from build123d import *

# Parameters (mm, degrees)
CROQUIS1_W              = 41
CROQUIS1_H              = 23.5
CROQUIS1_R              = 5.3
SALIENTE_EXTRUIR1_DEPTH = 3
CROQUIS3_W              = 41
CROQUIS3_H              = 3
SALIENTE_EXTRUIR2_DEPTH = 27
CROQUIS4_R              = 1.8
SALIENTE_EXTRUIR3_DEPTH = 3
CROQUIS5_W              = 8.5
CROQUIS5_H              = 3
SALIENTE_EXTRUIR4_DEPTH = 27
CROQUIS6_W              = 38
CROQUIS6_H              = 3
SALIENTE_EXTRUIR5_DEPTH = 12
CORTAR_EXTRUIR3_REACH   = 54.868
CROQUIS10_R             = 2.45
CROQUIS16_W             = 3
CROQUIS16_H             = 24
SALIENTE_EXTRUIR6_DEPTH = 1
CROQUIS17_W             = 3
CROQUIS17_H             = 24
SALIENTE_EXTRUIR7_DEPTH = 1
CORTAR_EXTRUIR1_REACH   = 47.167
CROQUIS8_R              = 5.3
CORTAR_EXTRUIR2_REACH   = 57.779
CROQUIS9_R              = 1.95
REDONDEO1_R             = 4
REDONDEO2_R             = 3
REDONDEO3_R             = 1
REDONDEO4_R             = 2
CROQUIS11_R             = 1.8
CORTAR_EXTRUIR4_DEPTH   = 5
CROQUIS12_R             = 1.8
CORTAR_EXTRUIR5_DEPTH   = 5
CROQUIS14_R             = 1.9
CORTAR_EXTRUIR6_DEPTH   = 5
CROQUIS15_W             = 6
CROQUIS15_H             = 3
CORTAR_EXTRUIR7_DEPTH   = 6
CHAFL_N1_SIZE           = 1


with BuildPart() as part:
    # Croquis1 → Saliente-Extruir1 (new body)
    with BuildSketch(Plane(origin=(0, 0, 0), x_dir=(1, 0, 0), z_dir=(0, 1, 0))):
        Rectangle(CROQUIS1_W, CROQUIS1_H)
        with Locations(Location((0, 1.15, 0), (0, 0, 270))):
            Circle(CROQUIS1_R, mode=Mode.SUBTRACT)
    extrude(amount=SALIENTE_EXTRUIR1_DEPTH)

    # Croquis3 → Saliente-Extruir2 (add)
    with BuildSketch(Plane.XZ):
        with Locations((0, -13.25)):
            Rectangle(CROQUIS3_W, CROQUIS3_H)
    extrude(amount=-SALIENTE_EXTRUIR2_DEPTH)

    # Croquis4 → Saliente-Extruir3 (add)
    with BuildSketch(Plane.XZ):
        with BuildLine():
            Line((-20.5, -6.75), (-25, -6.75))
            ThreePointArc((-25, -6.75), (-27.828427125, -5.578427125), (-29, -2.75))
            Line((-29, -2.75), (-29, 17.25))
            Line((-29, 17.25), (-20.5, 17.25))
            Line((-20.5, 17.25), (-20.5, -6.75))
        make_face()
        with Locations(Location((-24.160816052, -1.62, 0), (0, 0, 270))):
            Circle(CROQUIS4_R, mode=Mode.SUBTRACT)
        with Locations(Location((-24.160816052, 8.38, 0), (0, 0, 270))):
            Circle(CROQUIS4_R, mode=Mode.SUBTRACT)
    saliente_extruir3 = extrude(amount=-SALIENTE_EXTRUIR3_DEPTH)

    # Croquis5 → Saliente-Extruir4 (add)
    with BuildSketch(Plane.XZ):
        with Locations((-24.75, 18.75)):
            Rectangle(CROQUIS5_W, CROQUIS5_H)
    saliente_extruir4 = extrude(amount=-SALIENTE_EXTRUIR4_DEPTH)

    # Croquis6 → Saliente-Extruir5 (add)
    with BuildSketch(Plane.XY.offset(11.75)):
        with Locations((0, 1.5)):
            Rectangle(CROQUIS6_W, CROQUIS6_H)
    extrude(amount=SALIENTE_EXTRUIR5_DEPTH)

    # Croquis10 → Cortar-Extruir3 (cut, up to next)
    with BuildSketch(Plane.XY.offset(20.25), mode=Mode.PRIVATE) as cortar_extruir3_sk1:
        with Locations((-24.25, 10.87)):
            Circle(CROQUIS10_R)
    cortar_extruir3_tool1 = extrude(cortar_extruir3_sk1.sketch, amount=-CORTAR_EXTRUIR3_REACH, mode=Mode.PRIVATE) & part.part
    # Croquis10 → Cortar-Extruir3 (cut, up to next)
    with BuildSketch(Plane.XY.offset(20.25), mode=Mode.PRIVATE) as cortar_extruir3_sk2:
        with Locations((-24.25, 20.87)):
            Circle(CROQUIS10_R)
    cortar_extruir3_tool2 = extrude(cortar_extruir3_sk2.sketch, amount=-CORTAR_EXTRUIR3_REACH, mode=Mode.PRIVATE) & part.part
    cortar_extruir3_1 = cortar_extruir3_tool1.solids().sort_by_distance((-24.25, 10.87, 20.25))[0]
    add(cortar_extruir3_1, mode=Mode.SUBTRACT)
    cortar_extruir3_2 = cortar_extruir3_tool2.solids().sort_by_distance((-24.25, 20.87, 20.25))[0]
    add(cortar_extruir3_2, mode=Mode.SUBTRACT)
    cortar_extruir3 = cortar_extruir3_1 + cortar_extruir3_2  # Cortar-Extruir3 as one shape, for the pattern or mirror that repeats it

    # Simetría3: Saliente-Extruir3, Saliente-Extruir4, Cortar-Extruir3 across plane
    add(saliente_extruir3.mirror(Plane(origin=(0, 0, 0), x_dir=(0, 0, 1), z_dir=(1, 0, 0))))
    add(saliente_extruir4.mirror(Plane(origin=(0, 0, 0), x_dir=(0, 0, 1), z_dir=(1, 0, 0))))
    add(cortar_extruir3.mirror(Plane(origin=(0, 0, 0), x_dir=(0, 0, 1), z_dir=(1, 0, 0))), mode=Mode.SUBTRACT)

    # Croquis16 → Saliente-Extruir6 (add)
    with BuildSketch(Plane(origin=(29, 0, 0), x_dir=(0, 0, -1), z_dir=(1, 0, 0))):
        with Locations((-18.75, 15)):
            Rectangle(CROQUIS16_W, CROQUIS16_H)
    extrude(amount=SALIENTE_EXTRUIR6_DEPTH)

    # Croquis17 → Saliente-Extruir7 (add)
    with BuildSketch(Plane.ZY.offset(29)):
        with Locations((18.75, 15)):
            Rectangle(CROQUIS17_W, CROQUIS17_H)
    extrude(amount=SALIENTE_EXTRUIR7_DEPTH)

    # Croquis8 → Cortar-Extruir1 (cut, up to next)
    with BuildSketch(Plane(origin=(0, 3, 0), x_dir=(1, 0, 0), z_dir=(0, 1, 0)), mode=Mode.PRIVATE) as cortar_extruir1_sk1:
        with Locations(Location((-9.75, -12.22, 0), (0, 0, 270))):
            Circle(CROQUIS8_R)
    cortar_extruir1_tool1 = extrude(cortar_extruir1_sk1.sketch, amount=-CORTAR_EXTRUIR1_REACH, mode=Mode.PRIVATE) & part.part
    cortar_extruir1 = cortar_extruir1_tool1.solids().sort_by_distance((-9.75, 3, 12.22))[0]
    add(cortar_extruir1, mode=Mode.SUBTRACT)

    # Simetría4: Cortar-Extruir1 across plane
    add(cortar_extruir1.mirror(Plane(origin=(0, 0, 0), x_dir=(0, 0, 1), z_dir=(1, 0, 0))), mode=Mode.SUBTRACT)

    # Croquis9 → Cortar-Extruir2 (cut, up to next)
    with BuildSketch(Plane(origin=(0, 0, -14.75), x_dir=(-1, 0, 0), z_dir=(0, 0, -1)), mode=Mode.PRIVATE) as cortar_extruir2_sk1:
        with Locations((-10, 15.87)):
            Circle(CROQUIS9_R)
    cortar_extruir2_tool1 = extrude(cortar_extruir2_sk1.sketch, amount=-CORTAR_EXTRUIR2_REACH, mode=Mode.PRIVATE) & part.part
    # Croquis9 → Cortar-Extruir2 (cut, up to next)
    with BuildSketch(Plane(origin=(0, 0, -14.75), x_dir=(-1, 0, 0), z_dir=(0, 0, -1)), mode=Mode.PRIVATE) as cortar_extruir2_sk2:
        with Locations((10, 15.87)):
            Circle(CROQUIS9_R)
    cortar_extruir2_tool2 = extrude(cortar_extruir2_sk2.sketch, amount=-CORTAR_EXTRUIR2_REACH, mode=Mode.PRIVATE) & part.part
    add(cortar_extruir2_tool1.solids().sort_by_distance((10, 15.87, -14.75))[0], mode=Mode.SUBTRACT)
    add(cortar_extruir2_tool2.solids().sort_by_distance((-10, 15.87, -14.75))[0], mode=Mode.SUBTRACT)

    # Redondeo1
    redondeo1_edges = [part.edges().sort_by_distance(p)[0] for p in [
        (-19, 1.5, 23.75),
        (19, 1.5, 23.75),
        (20.5, 27, -13.25),
        (-20.5, 27, -13.25),
        (-30, 27, 18.75),
        (30, 27, 18.75),
    ]]
    fillet(redondeo1_edges, radius=REDONDEO1_R)

    # Redondeo2
    redondeo2_edges = [part.edges().sort_by_distance(p)[0] for p in [
        (24.75, 0, 20.25),
        (0, 0, -14.75),
        (-24.75, 0, 20.25),
    ]]
    fillet(redondeo2_edges, radius=REDONDEO2_R)

    # Redondeo3
    redondeo3_edges = [part.edges().sort_by_distance(p)[0] for p in [
        (0, 3, -11.75),
    ]]
    fillet(redondeo3_edges, radius=REDONDEO3_R)

    # Redondeo4
    redondeo4_edges = [part.edges().sort_by_distance(p)[0] for p in [
        (24.75, 3, 17.25),
        (-24.75, 3, 17.25),
    ]]
    fillet(redondeo4_edges, radius=REDONDEO4_R)

    # Croquis11 → Cortar-Extruir4 (cut)
    with BuildSketch(Plane(origin=(0, 0, 0), x_dir=(1, 0, 0), z_dir=(0, 1, 0))):
        with Locations((7.424621202, -6.274621202)):
            Circle(CROQUIS11_R)
        with Locations((-7.424621202, -6.274621202)):
            Circle(CROQUIS11_R)
        with Locations(Location((-7.424621202, 8.574621202, 0), (0, 0, 270))):
            Circle(CROQUIS11_R)
        with Locations(Location((7.424621202, 8.574621202, 0), (0, 0, 270))):
            Circle(CROQUIS11_R)
    extrude(amount=CORTAR_EXTRUIR4_DEPTH, mode=Mode.SUBTRACT)

    # Croquis12 → Cortar-Extruir5 (cut)
    with BuildSketch(Plane.XZ):
        with Locations(Location((-2.325378798, 19.644621202, 0), (0, 0, 270))):
            Circle(CROQUIS12_R)
        with Locations((-2.325378798, 4.795378798)):
            Circle(CROQUIS12_R)
        with Locations(Location((-17.174621202, 4.795378798, 0), (0, 0, 270))):
            Circle(CROQUIS12_R)
        with Locations(Location((-17.174621202, 19.644621202, 0), (0, 0, 270))):
            Circle(CROQUIS12_R)
    extrude(amount=-CORTAR_EXTRUIR5_DEPTH, mode=Mode.SUBTRACT)

    # Croquis14 → Cortar-Extruir6 (cut)
    with BuildSketch(Plane.XZ):
        with Locations((17.174621202, 19.644621202)):
            Circle(CROQUIS14_R)
        with Locations(Location((17.174621202, 4.795378798, 0), (0, 0, 270))):
            Circle(CROQUIS14_R)
        with Locations((2.325378798, 4.795378798)):
            Circle(CROQUIS14_R)
        with Locations(Location((2.325378798, 19.644621202, 0), (0, 0, 270))):
            Circle(CROQUIS14_R)
    extrude(amount=-CORTAR_EXTRUIR6_DEPTH, mode=Mode.SUBTRACT)

    # Croquis15 → Cortar-Extruir7 (cut)
    with BuildSketch(Plane(origin=(0, 0, -14.75), x_dir=(-1, 0, 0), z_dir=(0, 0, -1))):
        with Locations((-0.0498677, 4.5)):
            Rectangle(CROQUIS15_W, CROQUIS15_H)
    extrude(amount=-CORTAR_EXTRUIR7_DEPTH, mode=Mode.SUBTRACT)

    # Chaflán1
    # the kernel refuses this chamfer: 1 mm, written as the material it adds along each edge
    with BuildSketch(Plane(origin=(29, 3, 22.821682988), x_dir=(-0.02749587661058563, -0.9996219169112968, 0), z_dir=(0, 0, -1))) as chafl_n1_piece_1_section:
        Polygon((CHAFL_N1_SIZE * 0.999621916911, -CHAFL_N1_SIZE * 0.0274958766106), (-CHAFL_N1_SIZE * 0.0274958766106, -CHAFL_N1_SIZE * 0.999621916911), (0, 0), align=None)
    chafl_n1_piece_1 = extrude(amount=5.571682988, mode=Mode.PRIVATE)
    chafl_n1_piece_1 = chafl_n1_piece_1 & Plane(origin=(29.334600076, 3, 17.25), x_dir=(0, -1, 0), z_dir=(1, 0, 0)) * Cylinder(3, 16, mode=Mode.PRIVATE)
    add(chafl_n1_piece_1)
    with BuildSketch(Plane(origin=(-29, 3, 22.821682988), x_dir=(0.02749587661058563, -0.9996219169112968, 0), z_dir=(0, 0, -1))) as chafl_n1_piece_2_section:
        Polygon((CHAFL_N1_SIZE * 0.999621916911, CHAFL_N1_SIZE * 0.0274958766106), (-CHAFL_N1_SIZE * 0.0274958766106, CHAFL_N1_SIZE * 0.999621916911), (0, 0), align=None)
    chafl_n1_piece_2 = extrude(amount=5.571682988, mode=Mode.PRIVATE)
    chafl_n1_piece_2 = chafl_n1_piece_2 & Plane(origin=(-29.334600076, 3, 17.25), x_dir=(0, -1, 0), z_dir=(-1, 0, 0)) * Cylinder(3, 16, mode=Mode.PRIVATE)
    add(chafl_n1_piece_2)


solid = part.part
Read the model definition and answer for the solid it produces. Units are mm, in the model's axes. A direction names the side the tool comes from. Round coordinates to 2 decimals unless told otherwise and drop trailing zeros. Order: outer loops, then holes, each group sorted by start corner. A loop starts at its lowest first (then second) coordinate and runs counter-clockwise, first axis right, second up. Notation, with made-up numbers: (50, 15) - (92, 15) arc R12 cw to (92, 35) - close; hole circle Ø6 at (86, 27.5). An arc over 180 degrees is marked (long way). Use one line per item in the form item = value. Start each with the question number.
(1) Find the intervals of material crossed by line 1 along Y through (x, z) = (-24.25, 18.4); line 2 along Y through (x, z) = (-6.5, -7); line 3 along Z through (x, y) = (26, 7.25), in increasing order. Write a range as from..to.
(2) Determine the mould class of faces 6 (the face through (22.376, 1.479, -1.386)), 7 (the face through (0.29, 0.86, -13.85)), 8 (the face through (19, 1, 15)), 9 (the face through (-19.359, 25.797, -13.229)) for opening direction X: +X half, -X half, draft (parallel to the pull), parting line (faces both ways), or undercut.
(3) Flat-ended cylindrical pins translate along their axes: pin 1 Ø7.5 at (x, y) = (-26.5, 15) entering from -Z; pin 2 Ø5 at (x, z) = (-20.5, 12.5) entering from +Y; pin 3 Ø1.5 at (x, y) = (-23.5, 1.5) entering from -Z; pin 4 Ø4 at (x, y) = (24.25, 20.87) entering from +Z. Find the tip coordinate at first contact, or state that the pin passes through.
(4) The part is cut by section A-A (y = 20.87). Give the vertices of the cut face in (x, z).
(5) The part is cut by section B-B (z = 11). Give the vertices of the cut face in (x, y).
(6) For faces 1 (the face through (-20, 1, 11.75)), 2 (the face through (25.32, 0.9, 19.39)), 3 (the face through (-25.32, 0.86, 19.35)), 4 (the face through (6.82, 1.48, 4.58)), 5 (the face through (0, 6, -13)), determine the directions among +Z, -Z, +X, -X, +Y, -Y from which every point of the face is accessible in a straight line to the end or side of a thin tool.
(7) The part is cut by section C-C (z = -1.15). Give the vertices of the cut face in (x, y), then the cut area to 3 significant figures.
(8) The part is cut by section D-D (x = -10). Give the vertices of the cut face in (y, z), then the cut area to 3 significant figures.
Checked values:
q1.line_1 = 0.23..8.42, 13.32..18.42, 23.32..27
q1.line_2 = 0..3
q1.line_3 = 17.25..20.25
q2.face_6 = undercut
q2.face_7 = draft
q2.face_8 = undercut
q2.face_9 = -X half
q3.pin_1 = 17.25
q3.pin_2 = 3
q3.pin_3 = -6.75
q3.pin_4 = through
q4.outline = (-30, 17.25) - (-26.7, 17.25) - (-26.7, 20.25) - (-30, 20.25) - close; (-21.8, 17.25) - (-20.5, 17.25) - (-20.5, 20.25) - (-21.8, 20.25) - close; (-20.5, -14.75) - (20.5, -14.75) - (20.5, -11.75) - (-20.5, -11.75) - close; (20.5, 17.25) - (21.8, 17.25) - (21.8, 20.25) - (20.5, 20.25) - close; (26.7, 17.25) - (30, 17.25) - (30, 20.25) - (26.7, 20.25) - close
q5.outline = (-29, 0) - (-14.91, 0) - (-14.91, 3) - (-29, 3) - close; (-4.59, 0) - (4.59, 0) - (4.59, 3) - (-4.59, 3) - close; (14.91, 0) - (29, 0) - (29, 3) - (14.91, 3) - close
q6.face_1 = +Z, +Y, -Y
q6.face_2 = +Z, +X, -Y
q6.face_3 = +Z, -X, -Y
q6.face_4 = +Y, -Y
q6.face_5 = +Z, -Z
q7.outline = (-29, 0) - (-25.9, 0) - (-25.9, 3) - (-29, 3) - close; (-22.42, 0) - (-5.3, 0) - (-5.3, 3) - (-22.42, 3) - close; (5.3, 0) - (22.42, 0) - (22.42, 3) - (5.3, 3) - close; (25.9, 0) - (29, 0) - (29, 3) - (25.9, 3) - close
q7.area = 121 mm^2
q8.outline = (0, -11.75) arc R3 ccw to (3, -14.75) - (13.92, -14.75) - (13.92, -11.75) - (4, -11.75) arc R1 cw to (3, -10.75) - (3, 6.93) - (0, 6.93) - close; (0, 17.51) - (3, 17.51) - (3, 23.75) - (0, 23.75) - close; (17.82, -14.75) - (27, -14.75) - (27, -11.75) - (17.82, -11.75) - close
q8.area = 142 mm^2
